Geometry check sheet. Reference: drawing and pictorial views, mm from the part's lowest x, y, z. Give positions to 0.01 mm unless a question says otherwise; leave off trailing zeros. Write each loop counter-clockwise with the first axis right and the second up, starting at its lowest first coordinate (ties: lowest second). Pieces come first, ordered by that corner, then holes. Notation, with made-up numbers: (87.5, -5.75) -> (91.5, -5.75) arc R3 cw to (91.5, -1.75) -> close; hole circle Ø8 at (5, 68.5). An arc over 180 degrees is marked (long way). Use a Markdown table: item, result. Add a question column.
1. Gauge pin test, flat end, axial feed: P1, Ø5.5, axis at x = 12.7, y = 12.7, coming from the -Z side. Record the tip position at first contact, or that the pin passes through.
2. Cross-section at B-B (z = 1.8). Count the separate pieces of the cut face and the enclosed holes in it, then the cut area to 3 significant figures.
3. Cross-section at A-A (y = 12.7). Enter the section's corners in (x, z) (1 decimal), then the cut area to 3 significant figures.
4. Scan lines: probe 1 along X at (y, z) = (12.7, 2.55) (1 decimal); probe 2 along X at (y, z) = (33.5, 2.6); probe 3 along X at (y, z) = (10, 1.9). Record each from-to range of solid material in increasing order. Write a range as [from, to].
5. Cross-section at D-D (x = 15). Enter the section's corners in (y, z) (1 decimal), then the cut area to 3 significant figures.
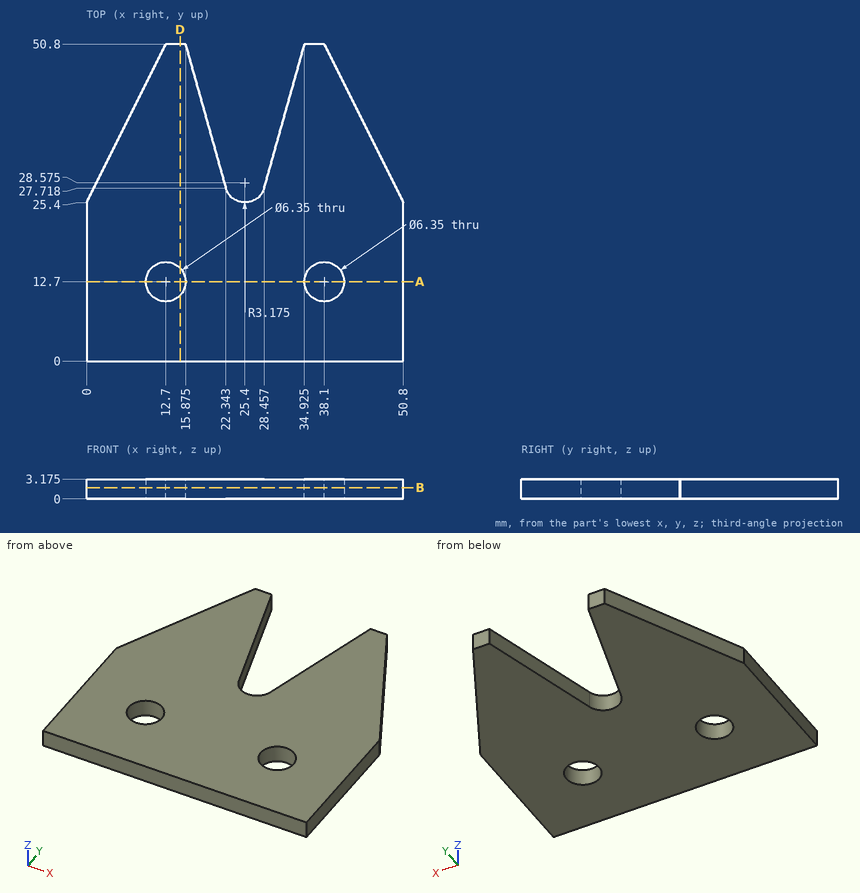
Worked answers:
| question | item | result |
|---|---|---|
| 1 | P1 | passes through |
| 2 | separate pieces | 1 |
| 2 | enclosed holes | 2 |
| 2 | area | 1,890 mm² |
| 3 | outline | (0, 0) -> (9.5, 0) -> (9.5, 3.2) -> (0, 3.2) -> close; (15.9, 0) -> (34.9, 0) -> (34.9, 3.2) -> (15.9, 3.2) -> close; (41.3, 0) -> (50.8, 0) -> (50.8, 3.2) -> (41.3, 3.2) -> close |
| 3 | area | 121 mm² |
| 4 | probe 1 | x = [0, 9.5], [15.9, 34.9], [41.3, 50.8] |
| 4 | probe 2 | x = [4.05, 20.72], [30.08, 46.75] |
| 4 | probe 3 | x = [0, 11.03], [14.37, 36.43], [39.77, 50.8] |
| 5 | outline | (0, 0) -> (10.5, 0) -> (10.5, 3.2) -> (0, 3.2) -> close; (14.9, 0) -> (50.8, 0) -> (50.8, 3.2) -> (14.9, 3.2) -> close |
| 5 | area | 147 mm² |
